```python
from build123d import *

# Parameters (mm, degrees)
SKETCH3_R      = 9.525
EXTRUDE1_DEPTH = 19.05


with BuildPart() as part:
    # Sketch3 → Extrude1 (new body)
    with BuildSketch(Plane.XY):
        with BuildLine():
            Line((0, 0), (101.6, 0))
            Line((101.6, 0), (101.6, 254))
            ThreePointArc((101.6, 254), (49.523585695, 379.723585695), (-76.2, 431.8))
            Line((-76.2, 431.8), (-203.2, 431.8))
            Line((-203.2, 431.8), (-203.2, 330.2))
            Line((-203.2, 330.2), (-76.2, 330.2))
            ThreePointArc((-76.2, 330.2), (-22.318463274, 307.881536726), (0, 254))
            Line((0, 254), (0, 0))
        make_face()
        with Locations((-177.8, 381)):
            Circle(SKETCH3_R, mode=Mode.SUBTRACT)
    extrude(amount=EXTRUDE1_DEPTH)


solid = part.part
```
The listing builds one solid part. Answer for the finished solid, in the listing's coordinates (mm). A direction names the side the tool comes from. Give positions to 0.01 mm unless a question says otherwise; leave off trailing zeros. Order: outer loops, then holes, each group sorted by start corner. A loop starts at its lowest first (then second) coordinate and runs counter-clockwise, first axis right, second up. Notation, with made-up numbers: M -29,31.5 L -8,31.5 A25 cw -8,54.5 Z; hole C 76.5,42 d6. An arc over 180 degrees is marked long. Put each result on its own line as item: value. Start each with the question number.
Item 1: For a pull along X with two mould halves and no side action, classify faces 3 (the face through (50, 0, 9)), 4 (the face through (50.9, 378.33, 9.39)), 5 (the face through (-179.86, 371.7, 9.39)) as +X half, -X half, draft (parallel to the pull), parting line (faces both ways), or undercut.
Item 2: The part is cut by section A-A, the plane x = -177.8. Determine the outline of the cut face in (y, z) (3 decimals).
Item 3: Which of the six approach directions +Z, -Z, +X, -X, +Y, -Y give full straight-line access (tool end or side, diameter ignored) to faces 1 (the face through (15, 267, 19.05)), 2 (the face through (-141, 330.2, 9))?
Item 4: Flat-ended cylindrical pins translate along their axes: P1, Ø2, axis at x = -60, z = 16.5, coming from the +Y side; P2, Ø5, axis at x = -89, z = 14, coming from the -Y side; P3, Ø1.5, axis at x = -58, y = 344.5, coming from the -Z side; P4, Ø5, axis at y = 249, z = 6, coming from the -X side. Find the tip coordinate at first contact, or state that the pin passes through.
Item 5: Find the intervals of material crossed by line 1 along Y through (x, z) = (-177.8, 5.5) (3 decimals); line 2 along X through (y, z) = (199, 16.25); line 3 along Y through (x, z) = (-121.5, 16.75), in increasing order.
Item 6: The part is cut by section B-B, the plane z = 10.75. Determine the outline of the cut face in (x, y) (3 decimals).
Item 7: The part is cut by section D-D, the plane y = 241. Determine the outline of the cut face in (x, z).
Item 8: The part is cut by section C-C, the plane y = 381. Determine the outline of the cut face in (x, z) (3 decimals), and give its area (3 significant figures).
Answer key:
1. face 3: draft
1. face 4: +X half
1. face 5: undercut
2. outline: M 330.2,0 L 371.475,0 L 371.475,19.05 L 330.2,19.05 Z; M 390.525,0 L 431.8,0 L 431.8,19.05 L 390.525,19.05 Z
3. face 1: +Z, +X, -X, +Y, -Y
3. face 2: +Z, -Z, -X, -Y
4. P1: stops at y = 431.15
4. P2: stops at y = 330.2
4. P3: stops at z = 0
4. P4: stops at x = 0
5. line 1: y = 330.2 to 371.475, 390.525 to 431.8
5. line 2: x = 0 to 101.6
5. line 3: y = 330.2 to 431.8
6. outline: M -203.2,330.2 L -76.2,330.2 A76.2 cw 0,254 L 0,0 L 101.6,0 L 101.6,254 A177.8 ccw -76.2,431.8 L -203.2,431.8 Z; hole C -177.8,381 d19.05
7. outline: M 0,0 L 101.6,0 L 101.6,19.05 L 0,19.05 Z
8. outline: M -203.2,0 L -187.325,0 L -187.325,19.05 L -203.2,19.05 Z; M -168.275,0 L 48.234,0 L 48.234,19.05 L -168.275,19.05 Z
8. area: 4,430 mm²
